Solid Edge part; units mm, degrees
sketch "Sketch1" plane through (0, 0, 0) normal (0, 0, 1) x (1, 0, 0)
  circle A0 centre (0, 0) radius 17.5
extrude "Protrusion1" add sketch "Sketch1" against normal blind 240
fillet "Redondeo_3" radius 10 1 edges at (-17.5, 0, -240)
sketch "Sketch2" plane through (0, 0, 0) normal (0, 0, 1) x (0, 1, 0)
  circle A0 centre (0, 0) radius 16.5
extrude "VaciadoExtruido_2" cut sketch "Sketch2" against normal blind 230
properties material "Cristal, industrial"
Input: part model. Units: mm. Frame: model coordinates. Round coordinates to 2 decimals unless told otherwise and drop trailing zeros. Loops run counter-clockwise (first coordinate to the right, second up) from the corner with the lowest first, then second, coordinate; pieces in that order, holes last. Notation, with made-up numbers: (-27.5, 55.5) -> (-12.5, 55.5) arc R21 ccw to (-12.5, 68.5) -> close; hole circle Ø8 at (-10.75, 47.25). An arc over 180 degrees is marked (long way). Use one line per item in the form item = value. Start each with the question number.
Item 1: Material intervals for L1, parallel to Y at x = 0, z = -103.5; L2, parallel to X at y = -1, z = -132.5; L3, parallel to Y at x = -9.5, z = -130, sorted ascending. Write a range as from..to.
Item 2: Contact query for flat-ended pins moving along their axis: pin 1 Ø4 at (y, z) = (-2.5, -52) entering from -X; pin 2 Ø10 at (x, y) = (6.5, 8) entering from +Z; pin 3 Ø6 at (y, z) = (-14, -150.5) entering from +X. Output: stop coordinate, or through.
Item 3: Mould query, pull axis X, two halves, no side actions, for faces 1 (the face through (-13.887, -10.648, -113.39)), 2 (the face through (6.32, 15.24, -113.39)), 3 (the face through (0, 0, -230)), 4 (the face through (0, 0, -240)). Classes: pulls with the +X half, pulls with the -X half, needs draft (parallel to the pull), parting line crosses it, or undercut.
Item 4: Section query A-A on z = -119. Return the cut outline in (x, y), then the cut area to 3 significant figures.
Ans:
q1.L1 = -17.5..-16.5, 16.5..17.5
q1.L2 = -17.47..-16.47, 16.47..17.47
q1.L3 = -14.7..-13.49, 13.49..14.7
q2.pin_1 = -17.49
q2.pin_2 = -230
q2.pin_3 = 13.61
q3.face_1 = parting line crosses it
q3.face_2 = undercut
q3.face_3 = undercut
q3.face_4 = needs draft
q4.outline = circle Ø35 at (0, 0); hole circle Ø33 at (0, 0)
q4.area = 107 mm^2
